CAD build for the part. Positions are in the model's coordinates, mm. Face numbers are marked on the shaded views. Round coordinates to 2 decimals unless told otherwise and drop trailing zeros. Order: outer loops, then holes, each group sorted by start corner. A loop starts at its lowest first (then second) coordinate and runs counter-clockwise, first axis right, second up. Notation, with made-up numbers: (11, -18) - (51, -18) arc R19 ccw to (51, -6) - close; hole circle Ø11 at (74, 62.25). An arc over 180 degrees is marked (long way). Write item = value, one per line.
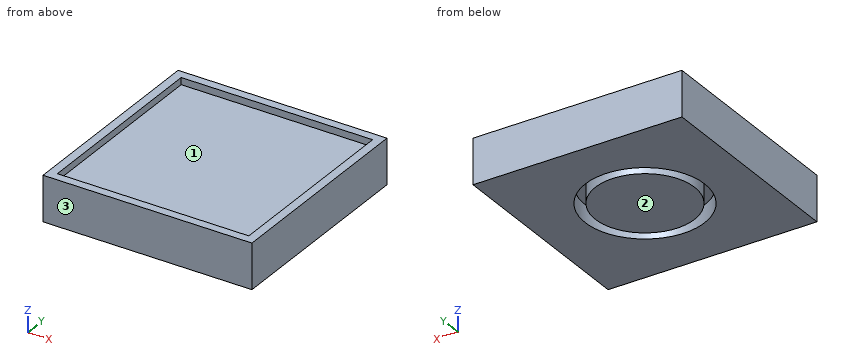
Autodesk Inventor part; units mm, degrees
ref_plane "YZ Plane" through (0, 0, 0) normal (1, 0, 0) x (0, 1, 0)
ref_plane "XZ Plane" through (0, 0, 0) normal (0, 1, 0) x (-1, 0, 0)
ref_plane "XY Plane" through (0, 0, 0) normal (0, 0, 1) x (1, 0, 0)
sketch "Sketch1" plane through (0, 0, 0) normal (0, 0, 1) x (1, 0, 0)
  line L0 (0, 0) -> (-150, 0)
  line L1 (-150, 0) -> (-150, 95)
  line L2 (-150, 95) -> (0, 95)
  line L3 (0, 95) -> (0, 0)
  dimension "d0" = 150
  dimension "d1" = 95
extrude "Extrusion1" add sketch "Sketch1" along normal blind 15
sketch "Sketch2" plane through (0, 0, 15) normal (0, 0, 1) x (1, 0, 0)
  line L0 (-32.5, 5) -> (-117.5, 5)
  line L1 (-117.5, 5) -> (-117.5, 90)
  line L2 (-117.5, 90) -> (-32.5, 90)
  line L3 (-32.5, 90) -> (-32.5, 5)
  point P0 (0, 0)
  dimension "d4" = 85
  dimension "d5" = 85
extrude "Extrusion2" cut sketch "Sketch2" against normal blind 2
sketch "Sketch3" plane through (0, 0, 13) normal (0, 0, 1) x (1, 0, 0)
  line L0 (-47.5, 75) -> (-102.5, 75)
  line L1 (-102.5, 75) -> (-102.5, 20)
  line L2 (-102.5, 20) -> (-47.5, 20)
  line L3 (-47.5, 20) -> (-47.5, 75)
  point P0 (0, 0)
  point P1 (-47.5, 47.5)
  dimension "d10" = 55
  dimension "d11" = 55
extrude "Extrusion3" cut sketch "Sketch3" against normal blind 2
sketch "Sketch4" plane through (0, 0, 0) normal (0, 0, -1) x (-1, 0, 0)
  circle A0 centre (75, 47.5) radius 14.25
  circle A1 centre (75, 47.5) radius 17.15
  line L0 (2.5, 2.5) -> (7.5, 2.5)
  line L1 (7.5, 2.5) -> (7.5, 7.5)
  line L2 (7.5, 7.5) -> (2.5, 7.5)
  line L3 (2.5, 7.5) -> (2.5, 2.5)
  line L4 (147.5, 2.5) -> (142.5, 2.5)
  line L5 (142.5, 2.5) -> (142.5, 7.5)
  line L6 (142.5, 7.5) -> (147.5, 7.5)
  line L7 (147.5, 7.5) -> (147.5, 2.5)
  line L8 (2.5, 92.5) -> (7.5, 92.5)
  line L9 (7.5, 92.5) -> (7.5, 87.5)
  line L10 (7.5, 87.5) -> (2.5, 87.5)
  line L11 (2.5, 87.5) -> (2.5, 92.5)
  line L12 (147.5, 92.5) -> (142.5, 92.5)
  line L13 (142.5, 92.5) -> (142.5, 87.5)
  line L14 (142.5, 87.5) -> (147.5, 87.5)
  line L15 (147.5, 87.5) -> (147.5, 92.5)
  point P0 (0, 0)
  dimension "d14" = 28.5
  dimension "d15" = 34.3
  dimension "d16" = 5
  dimension "d17" = 5
  dimension "d18" = 5
  dimension "d19" = 5
  dimension "d20" = 5
  dimension "d21" = 5
  dimension "d22" = 5
  dimension "d23" = 5
extrude "Extrusion4" cut sketch "Sketch4" against normal blind 5
sketch "Sketch5" plane through (0, 0, 0) normal (0, 0, -1) x (-1, 0, 0)
  line L0 (105, 77.5) -> (45, 77.5)
  line L1 (45, 77.5) -> (45, 17.5)
  line L2 (45, 17.5) -> (105, 17.5)
  line L3 (105, 17.5) -> (105, 77.5)
  line L4 (150, 0) -> (0, 0)
  line L5 (150, 95) -> (150, 0)
  line L6 (0, 0) -> (150, 0)
  line L7 (150, 0) -> (150, 95)
  line L8 (150, 95) -> (0, 95)
  line L9 (0, 95) -> (0, 0)
  dimension "d28" = 60
  dimension "d29" = 60
  dimension "d30" = 150
  dimension "d31" = 95
extrude "Extrusion5" cut sketch "Sketch5" against normal blind 15
properties part number "Shoulder_Both_Marker_V1"
(1) Band-saw the part on B-B on y = 47.5. List the corners of the cut face in (x, z), plus the area to 3 significant figures.
Solved:
outline = (-105, 0) - (-92.15, 0) - (-92.15, 5) - (-89.25, 5) - (-89.25, 0) - (-60.75, 0) - (-60.75, 5) - (-57.85, 5) - (-57.85, 0) - (-45, 0) - (-45, 13) - (-47.5, 13) - (-47.5, 11) - (-102.5, 11) - (-102.5, 13) - (-105, 13) - close
area = 641 mm²
(2) Band-saw the part on D-D on z = 11.75. List the corners of the cut face in (x, y).
Solved:
outline = (-105, 17.5) - (-45, 17.5) - (-45, 77.5) - (-105, 77.5) - close; hole (-102.5, 20) - (-47.5, 20) - (-47.5, 75) - (-102.5, 75) - close
(3) Drop a flat-ended pin along its axis: pin 1 (1.5 mm diameter, centred on x = -77.5, y = 66.5, fed in from +Z). Give the stop position or say it passes through.
Solved:
pin_1 = 11
(4) Probe line 1 along Y through (x, z) = (-75, 3.05); line 2 along Y through (x, z) = (-95.5, 11.5); line 3 along X through (y, z) = (22.5, 11.5). List the from-to ranges inside material, lowest first.
Solved:
line_1 = 17.5 to 30.35, 33.25 to 61.75, 64.65 to 77.5
line_2 = 17.5 to 20, 75 to 77.5
line_3 = -105 to -102.5, -47.5 to -45
(5) Band-saw the part on A-A on z = 1.25. List the corners of the cut face in (x, y).
Solved:
outline = (-105, 17.5) - (-45, 17.5) - (-45, 77.5) - (-105, 77.5) - close; circle Ø28.5 at (-75, 47.5); hole circle Ø34.3 at (-75, 47.5)
(6) Band-saw the part on C-C on x = -75. List the corners of the cut face in (y, z).
Solved:
outline = (17.5, 0) - (30.35, 0) - (30.35, 5) - (33.25, 5) - (33.25, 0) - (61.75, 0) - (61.75, 5) - (64.65, 5) - (64.65, 0) - (77.5, 0) - (77.5, 13) - (75, 13) - (75, 11) - (20, 11) - (20, 13) - (17.5, 13) - close
(7) Pull direction Y, two halves, no side cores. Call the marked faces 1, 2 and 3: released by +Y, released by -Y, zero draft, split by the parting line, or undercut.
Solved:
face_1 = undercut
face_2 = zero draft
face_3 = released by -Y
